from build123d import *

# Parameters (mm, degrees)
BOSS_EXTRUDE1_DEPTH = 12
SKETCH4_W           = 39.051681067
SKETCH4_H           = 24
SKETCH4_R           = 4
BOSS_EXTRUDE2_DEPTH = 12
SKETCH4_3_R         = 8
SKETCH4_3_R_2       = 4
CUT_EXTRUDE1_DEPTH  = 5.15
FILLET1_R           = 12
SKETCH5_R           = 1.7
CUT_EXTRUDE2_DEPTH  = 107.997244305
CUT_EXTRUDE3_START  = -5
SKETCH5_3_R         = 3
CUT_EXTRUDE3_DEPTH  = 102.997244335


with BuildPart() as part:
    # Sketch3 → Boss-Extrude1 (new body)
    with BuildSketch(Plane(origin=(0, 0, 0), x_dir=(1, 0, 0), z_dir=(0, 1, 0))):
        with BuildLine():
            Line((-4.215390309, -12), (-17.23368794, -12))
            ThreePointArc((-17.23368794, -12), (0, -21), (17.23368794, -12))
            Line((17.23368794, -12), (4.215390309, -12))
            Line((4.215390309, -12), (0, -14.43375673))
            Line((0, -14.43375673), (-4.215390309, -12))
        make_face()
        with BuildLine():
            Line((17.23368794, 12), (4.215390309, 12))
            Line((4.215390309, 12), (12.5, 7.216878365))
            Line((12.5, 7.216878365), (12.5, -7.216878365))
            Line((12.5, -7.216878365), (4.215390309, -12))
            Line((4.215390309, -12), (17.23368794, -12))
            ThreePointArc((17.23368794, -12), (20.036310124, -6.288583039), (21, 0))
            ThreePointArc((21, 0), (20.036310124, 6.288583039), (17.23368794, 12))
        make_face()
        with BuildLine():
            Line((-12.5, 7.216878365), (-4.215390309, 12))
            Line((-4.215390309, 12), (-17.23368794, 12))
            ThreePointArc((-17.23368794, 12), (-21, 0), (-17.23368794, -12))
            Line((-17.23368794, -12), (-4.215390309, -12))
            Line((-4.215390309, -12), (-12.5, -7.216878365))
            Line((-12.5, -7.216878365), (-12.5, 7.216878365))
        make_face()
        with BuildLine():
            Line((-4.215390309, 12), (0, 14.43375673))
            Line((0, 14.43375673), (4.215390309, 12))
            Line((4.215390309, 12), (17.23368794, 12))
            ThreePointArc((17.23368794, 12), (0, 21), (-17.23368794, 12))
            Line((-17.23368794, 12), (-4.215390309, 12))
        make_face()
        with BuildLine():
            Line((74.2, 12), (17.23368794, 12))
            ThreePointArc((17.23368794, 12), (20.036310124, 6.288583039), (21, 0))
            ThreePointArc((21, 0), (20.036310124, -6.288583039), (17.23368794, -12))
            Line((17.23368794, -12), (74.2, -12))
            Line((74.2, -12), (74.2, 12))
        make_face()
    extrude(amount=BOSS_EXTRUDE1_DEPTH)

    # Sketch4 → Boss-Extrude2 (add)
    with BuildSketch(Plane(origin=(37.1, -37.1, 0), x_dir=(0.7071067811865462, 0.7071067811865489, 0), z_dir=(0.7071067811865489, -0.7071067811865462, 0))):
        with Locations((71.993163698, 0)):
            Rectangle(SKETCH4_W, SKETCH4_H)
        with Locations((75.519004231, 0)):
            Circle(SKETCH4_R, mode=Mode.SUBTRACT)
    extrude(amount=-BOSS_EXTRUDE2_DEPTH)

    # Sketch4<3> → Cut-Extrude1 (cut)
    with BuildSketch(Plane(origin=(37.1, -37.1, 0), x_dir=(0.7071067811865462, 0.7071067811865489, 0), z_dir=(0.7071067811865489, -0.7071067811865462, 0))):
        with Locations((75.519004231, 0)):
            Circle(SKETCH4_3_R)
        with Locations((75.519004231, 0)):
            Circle(SKETCH4_3_R_2, mode=Mode.SUBTRACT)
    extrude(amount=-CUT_EXTRUDE1_DEPTH, mode=Mode.SUBTRACT)

    # Fillet1
    fillet1_edges = [part.edges().sort_by_distance(p)[0] for p in [
        (97.571067812, 31.856349186, -12),
        (97.571067812, 31.856349186, 12),
    ]]
    fillet(fillet1_edges, radius=FILLET1_R - 0.0001)  # a hair under: the kernel refuses the full size

    # Sketch5 → Cut-Extrude2 (cut, through all)
    with BuildSketch(Plane(origin=(6.25, 0, -10.825317547), x_dir=(0.8660254037844386, 0, 0.5), z_dir=(-0.5000000000000001, 0, 0.8660254037844387))):
        with Locations((0, 6)):
            Circle(SKETCH5_R)
    cut_extrude2 = extrude(amount=-CUT_EXTRUDE2_DEPTH, mode=Mode.SUBTRACT)

    # Sketch5<3> → Cut-Extrude3 (cut, through all)
    with BuildSketch(Plane(origin=(6.25, 0, -10.825317547), x_dir=(0.8660254037844386, 0, 0.5), z_dir=(-0.5000000000000001, 0, 0.8660254037844387)).offset(CUT_EXTRUDE3_START)):
        with Locations((0, 6)):
            Circle(SKETCH5_3_R)
    cut_extrude3 = extrude(amount=-CUT_EXTRUDE3_DEPTH, mode=Mode.SUBTRACT)

    # Mirror1: Cut-Extrude2, Cut-Extrude3 across plane
    add(cut_extrude2.mirror(Plane(origin=(0, 0, 0), x_dir=(0.8660254037844386, 0, 0.5000000000000002), z_dir=(-0.5, 0, 0.8660254037844386))), mode=Mode.SUBTRACT)
    add(cut_extrude3.mirror(Plane(origin=(0, 0, 0), x_dir=(0.8660254037844386, 0, 0.5000000000000002), z_dir=(-0.5, 0, 0.8660254037844386))), mode=Mode.SUBTRACT)


solid = part.part
Design review of the part built by this model. Coordinates are the model's own, in mm. A direction names the side the tool comes from. Round coordinates to 2 decimals unless told otherwise and drop trailing zeros. Write each loop counter-clockwise with the first axis right and the second up, starting at its lowest first coordinate (ties: lowest second). Pieces come first, ordered by that corner, then holes.
Item 1: Wall thickness on L1, parallel to Y at x = 36.5, z = -9; L2, parallel to X at y = 8, z = -10.5; L3, parallel to Y at x = 12, z = -17: over which ranges is each line inside the solid? List them lowest first.
Item 2: For faces 1 (the flat face through (-12.5, 6, 0)), 2 (the flat face through (23, 12, 0)), 3 (the flat face through (8.71, 4.04, -15.18)), 4 (the flat face through (84.7, 10.5, 0.2)), list the 3-axis set-ups (+Z, -Z, +X, -X, +Y, -Y) from which the entire face can be reached by the end or side of a thin tool; tool diameter is ignored.
Item 3: Consider section A-A on z = 2.5. Give the boundary of the cut face in (x, y), and give its area (3 significant figures).
Item 4: Draft analysis for pull direction X (two halves, no side actions). For faces 5 (the flat face through (55, 10, -12)), 6 (the cylindrical face through (8.2, 4.5, -12.6)), 7 (the flat face through (-8.786, 4.042, 15.134)), 8 (the cylindrical face through (94.96, 29.36, 8.58)), state which applies: released by +X, released by -X, zero draft, split by the parting line, or undercut.
Item 5: Consider section B-B on x = 45.5. Give the boundary of the cut face in (y, z).
Item 6: Consider section C-C on x = 70.5. Give the boundary of the cut face in (y, z), and give its area (3 significant figures).
Item 7: For pin 1 Ø13 at (y, z) = (7.5, 0) entering from -X; pin 2 Ø6 at (y, z) = (9, -3) entering from +X; pin 3 Ø8.5 at (x, y) = (40, 9) entering from -Z, all flat-tipped, find the tip position at first contact; note any pin that passes through.
Check values:
1. L1: y = 0 to 12
1. L2: x = -18.19 to -6.81, 6.81 to 82.2
1. L3: y = 0 to 3.67, 8.33 to 12
2. face 1: +Y, -Y
2. face 2: +Z, -Z, -X, +Y
2. face 3: none
2. face 4: +Z, -Z, +X, -Y
3. outline: (-20.85, 0) - (-12.5, 0) - (-12.5, 12) - (-20.85, 12) - close; (12.5, 0) - (74.2, 0) - (85.13, 10.93) - (81.48, 14.57) - (84.65, 17.73) - (79.81, 22.58) - (69.23, 12) - (12.5, 12) - close; (84.22, 26.99) - (89.07, 22.15) - (92.23, 25.32) - (95.87, 21.67) - (101.63, 27.43) - (93.14, 35.91) - close
3. area: 1,130 mm2
4. face 5: zero draft
4. face 6: undercut
4. face 7: undercut
4. face 8: released by +X
5. outline: (0, -12) - (12, -12) - (12, 12) - (0, 12) - close
6. outline: (0, -12) - (13.27, -12) - (13.27, 12) - (0, 12) - close
6. area: 318 mm2
7. pin 1: stops at x = -21
7. pin 2: stops at x = 85.81
7. pin 3: stops at z = -12
